```python
from build123d import *

# Parameters (mm, degrees)
SKETCH1_R           = 8
SKETCH1_R_2         = 3.125
BOSS_EXTRUDE1_DEPTH = 14
SKETCH2_R           = 1.5
CUT_EXTRUDE1_DEPTH  = 9
CUT_EXTRUDE2_START  = -3.025
CUT_EXTRUDE2_DEPTH  = 2.25
CUT_EXTRUDE3_START  = 3.025
CUT_EXTRUDE3_DEPTH  = 2.25
SKETCH5_R           = 6.25
BOSS_EXTRUDE2_DEPTH = 11.63
SKETCH6_R           = 4.5
BOSS_EXTRUDE3_DEPTH = 9.25
SKETCH7_R           = 1.5
CUT_EXTRUDE4_DEPTH  = 8
CUT_EXTRUDE5_START  = -3
SKETCH8_R           = 1.5
CUT_EXTRUDE5_DEPTH  = 2.5
SKETCH9_W           = 2.25
SKETCH9_H           = 3.25
CUT_EXTRUDE6_DEPTH  = 2
CIRPATTERN1_COUNT   = 3
CIRPATTERN3_COUNT   = 2
CIRPATTERN3_ANGLE   = 90


with BuildPart() as part:
    # Sketch1 → Boss-Extrude1 (new body)
    with BuildSketch(Plane(origin=(0, 0, 0), x_dir=(1, 0, 0), z_dir=(0, 1, 0))):
        Circle(SKETCH1_R)
        Circle(SKETCH1_R_2, mode=Mode.SUBTRACT)
    extrude(amount=BOSS_EXTRUDE1_DEPTH)

    # Sketch2 → Cut-Extrude1 (cut, symmetric)
    with BuildSketch(Plane.XY):
        with Locations((0, 4.5)):
            Circle(SKETCH2_R)
    cut_extrude1 = extrude(amount=CUT_EXTRUDE1_DEPTH, both=True, mode=Mode.SUBTRACT)

    # Sketch3 → Cut-Extrude2 (cut)
    with BuildSketch(Plane.XY.offset(CUT_EXTRUDE2_START)):
        Polygon((-2.75, 2.91228676), (0, 1.324573519), (2.75, 2.91228676), (2.75, 0), (-2.75, 0), align=None)
        Polygon((2.75, 2.91228676), (-2.75, 2.91228676), (-2.75, 6.08771324), (0, 7.675426481), (2.75, 6.08771324), align=None)
        Polygon((0, 1.324573519), (2.75, 2.91228676), (-2.75, 2.91228676), align=None)
    extrude(amount=-CUT_EXTRUDE2_DEPTH, mode=Mode.SUBTRACT)

    # Sketch4 → Cut-Extrude3 (cut)
    with BuildSketch(Plane.XY.offset(CUT_EXTRUDE3_START)):
        Polygon((-2.75, 2.91228676), (0, 1.324573519), (2.75, 2.91228676), (2.75, 0), (-2.75, 0), align=None)
        Polygon((0, 1.324573519), (2.75, 2.91228676), (-2.75, 2.91228676), align=None)
        Polygon((2.75, 2.91228676), (-2.75, 2.91228676), (-2.75, 6.08771324), (0, 7.675426481), (2.75, 6.08771324), align=None)
    extrude(amount=CUT_EXTRUDE3_DEPTH, mode=Mode.SUBTRACT)

    # Sketch5 → Boss-Extrude2 (add)
    with BuildSketch(Plane(origin=(0, 14, 0), x_dir=(1, 0, 0), z_dir=(0, 1, 0))):
        Circle(SKETCH5_R)
    extrude(amount=BOSS_EXTRUDE2_DEPTH)

    # Sketch6 → Boss-Extrude3 (add)
    with BuildSketch(Plane(origin=(0, 25.63, 0), x_dir=(1, 0, 0), z_dir=(0, 1, 0))):
        Circle(SKETCH6_R)
    extrude(amount=BOSS_EXTRUDE3_DEPTH)

    # Sketch7 → Cut-Extrude4 (cut)
    with BuildSketch(Plane(origin=(0, 34.88, 0), x_dir=(1, 0, 0), z_dir=(0, 1, 0))):
        Circle(SKETCH7_R)
    extrude(amount=-CUT_EXTRUDE4_DEPTH, mode=Mode.SUBTRACT)

    # Sketch8 → Cut-Extrude5 (cut)
    with BuildSketch(Plane(origin=(0, 34.88, 0), x_dir=(1, 0, 0), z_dir=(0, 1, 0)).offset(CUT_EXTRUDE5_START)):
        with BuildLine():
            Line((2.75, -1.58771324), (0, -3.175426481))
            Line((0, -3.175426481), (-2.75, -1.58771324))
            Line((-2.75, -1.58771324), (-2.75, -3.561951712))
            ThreePointArc((-2.75, -3.561951712), (0, -4.5), (2.75, -3.561951712))
            Line((2.75, -3.561951712), (2.75, -1.58771324))
        make_face()
        Polygon((-2.75, -1.58771324), (2.75, -1.58771324), (0, -3.175426481), align=None)
        Polygon((-2.75, 1.58771324), (-2.75, -1.58771324), (2.75, -1.58771324), (2.75, 1.58771324), (0, 3.175426481), align=None)
        Circle(SKETCH8_R, mode=Mode.SUBTRACT)
    extrude(amount=-CUT_EXTRUDE5_DEPTH, mode=Mode.SUBTRACT)

    # Sketch9 → Cut-Extrude6 (cut)
    with BuildSketch(Plane(origin=(0, 34.88, 0), x_dir=(1, 0, 0), z_dir=(0, 1, 0))):
        with Locations((0, 4.5)):
            Rectangle(SKETCH9_W, SKETCH9_H)
    cut_extrude6 = extrude(amount=-CUT_EXTRUDE6_DEPTH, mode=Mode.SUBTRACT)

    # CirPattern1: Cut-Extrude6 ×3 about axis
    cirpattern1_axis = Axis((0, 0, 0), (0, 1, 0))
    for i in range(1, CIRPATTERN1_COUNT):
        add(cut_extrude6.rotate(cirpattern1_axis, i * 360 / CIRPATTERN1_COUNT), mode=Mode.SUBTRACT)

    # CirPattern3: Cut-Extrude1 ×2 about axis
    cirpattern3_axis = Axis((0, 0, 0), (0, 1, 0))
    for i in range(1, CIRPATTERN3_COUNT):
        add(cut_extrude1.rotate(cirpattern3_axis, i * CIRPATTERN3_ANGLE / (CIRPATTERN3_COUNT - 1)), mode=Mode.SUBTRACT)


solid = part.part
```
Input: part model. Units: mm. Frame: model coordinates. A direction names the side the tool comes from. Round coordinates to 2 decimals unless told otherwise and drop trailing zeros. Order: outer loops, then holes, each group sorted by start corner. A loop starts at its lowest first (then second) coordinate and runs counter-clockwise, first axis right, second up. Notation, with made-up numbers: (-24.75, 74.25) - (-7.75, 74.25) arc R18 cw to (-7.75, 107.25) - close; hole circle Ø9 at (64.25, 5.5). An arc over 180 degrees is marked (long way). Answer in a Markdown table with one row per item.
Item 1: Reachability of faces 1 (the cylindrical face through (5.96, 19.73, -1.88)), 2 (the cylindrical face through (-1.5, 4.57, -6.62)), 3 (the flat face through (2.75, 3, -4)), 4 (the flat face through (1.125, 34, -4)) from +Z, -Z, +X, -X, +Y, -Y: full face, straight path, thin tool, end or side. Return the list, or none.
Model answer:
| item | result |
|---|---|
| face 1 | +Y |
| face 2 | +Z, -Z |
| face 3 | -Y |
| face 4 | -Z, +Y |
Item 2: Line query: line 1 (Y direction, x = 6.6, z = 0); line 2 (Z direction, x = -2.5, y = 2) (3 decimals); line 3 (Y direction, x = 1.75, z = -0.25). Output: solid intervals per line, ascending.
Model answer:
| item | result |
|---|---|
| line 1 | y = 0 to 3, 6 to 14 |
| line 2 | z = -7.599 to -5.275, -3.025 to -1.875, 1.875 to 3.025, 5.275 to 7.599 |
| line 3 | y = 14 to 29.38, 31.88 to 34.88 |
Item 3: Section query C-C (z = 0). Give the number of separate pieces and of enclosed holes in the cut face, then the cut area to 3 significant figures.
Model answer:
| item | result |
|---|---|
| separate pieces | 3 |
| enclosed holes | 0 |
| area | 306 mm² |
Item 4: Mould query, pull axis Y, two halves, no side actions, for faces 5 (the flat face through (0, 31.88, 2)), 6 (the flat face through (-3, 32.88, 2)), 7 (the flat face through (2, 4, -3.025)). Classes: released by +Y, released by -Y, zero draft, split by the parting line, or undercut.
Model answer:
| item | result |
|---|---|
| face 5 | undercut |
| face 6 | released by +Y |
| face 7 | zero draft |
Item 5: Section query A-A (x = -5.5). Return the cut outline in (y, z).
Model answer:
| item | result |
|---|---|
| outline | (0, -5.81) - (14, -5.81) - (14, -2.97) - (25.63, -2.97) - (25.63, 2.97) - (14, 2.97) - (14, 5.81) - (0, 5.81) - close; hole circle Ø3 at (4.5, 0) |
Item 6: Section query B-B (y = 30.5). Return the cut outline in (x, z).
Model answer:
| item | result |
|---|---|
| outline | (-2.75, -1.59) - (-2.75, 3.56) arc R4.5 ccw (long way) to (2.75, 3.56) - (2.75, -1.59) - (0, -3.18) - close |
Item 7: Pin query (flat end, axial travel): pin 1 (3 mm diameter, centred on y = 16.5, z = 5, fed in from +X); pin 2 (6 mm diameter, centred on x = 0.5, z = -6, fed in from +Y); pin 3 (1.6 mm diameter, centred on x = 1.5, y = 4.5, fed in from +Z); pin 4 (3 mm diameter, centred on y = 31, z = 3, fed in from +X). Return the tip coordinate at first contact, or that it passes through.
Model answer:
| item | result |
|---|---|
| pin 1 | stops at x = 5.18 |
| pin 2 | stops at y = 34.88 |
| pin 3 | stops at z = 7.9 |
| pin 4 | stops at x = 4.24 |
